```python
from build123d import *

# Parameters (mm, degrees)
F0_W     = 126
F0_H     = 129
F0_R     = 4
F1_DEPTH = 5


with BuildPart() as f1:
    # F0 (on Front) → F1 (new body)
    with BuildSketch(Plane.XZ):
        with Locations((63, 64.5)):
            Rectangle(F0_W, F0_H)
        with Locations((17, 27.5)):
            Circle(F0_R, mode=Mode.SUBTRACT)
        with Locations((17, 52.5)):
            Circle(F0_R, mode=Mode.SUBTRACT)
        with Locations((109, 27.5)):
            Circle(F0_R, mode=Mode.SUBTRACT)
        with Locations((109, 52.5)):
            Circle(F0_R, mode=Mode.SUBTRACT)
        with Locations((22, 107.5)):
            Circle(F0_R, mode=Mode.SUBTRACT)
        Polygon((93, 19), (33, 19), (24, 28), (24, 90), (49, 115), (77, 115), (102, 90), (102, 28), align=None, mode=Mode.SUBTRACT)
        with Locations((104, 107.5)):
            Circle(F0_R, mode=Mode.SUBTRACT)
    extrude(amount=F1_DEPTH)


solid = f1.part
```
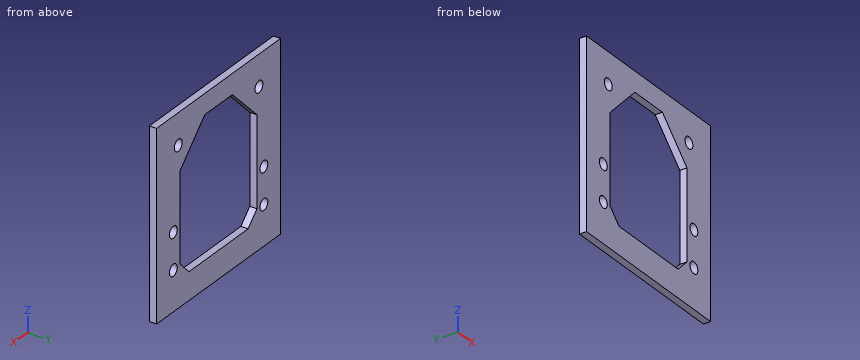
Design review of the part built by this model. Coordinates are the model's own, in mm. Round coordinates to 2 decimals unless told otherwise and drop trailing zeros. Write each loop counter-clockwise with the first axis right and the second up, starting at its lowest first coordinate (ties: lowest second). Pieces come first, ordered by that corner, then holes. Notation, with made-up numbers: (-2, -38.5) -> (53, -38.5) arc R18 ccw to (53, -18.5) -> close; hole circle Ø6 at (85.5, 11.5). An arc over 180 degrees is marked (long way). Answer in a Markdown table with one row per item.
Q1. To check wall thickness, follow L1, parallel to Z at x = 109, y = -2; L2, parallel to X at y = -2.15, z = 80.5; L3, parallel to Z at x = 36, y = -1.75. State the ranges of each line that lie inside material, in increasing order. Write a range as [from, to].
The answers:
| item | result |
|---|---|
| L1 | [0, 23.5], [31.5, 48.5], [56.5, 129] |
| L2 | [0, 24], [102, 126] |
| L3 | [0, 19], [102, 129] |
Q2. Take a section at D-D, the plane z = 38.5. State the section outline as (x, y) points, then the cut area to 3 significant figures.
The answers:
| item | result |
|---|---|
| outline | (0, -5) -> (24, -5) -> (24, 0) -> (0, 0) -> close; (102, -5) -> (126, -5) -> (126, 0) -> (102, 0) -> close |
| area | 240 mm² |
Q3. Take a section at B-B, the plane y = -0.9. State the section outline as (x, z) points.
The answers:
| item | result |
|---|---|
| outline | (0, 0) -> (126, 0) -> (126, 129) -> (0, 129) -> close; hole circle Ø8 at (17, 27.5); hole circle Ø8 at (17, 52.5); hole circle Ø8 at (22, 107.5); hole (24, 28) -> (33, 19) -> (93, 19) -> (102, 28) -> (102, 90) -> (77, 115) -> (49, 115) -> (24, 90) -> close; hole circle Ø8 at (104, 107.5); hole circle Ø8 at (109, 27.5); hole circle Ø8 at (109, 52.5) |
Q4. Take a section at A-A, the plane z = 107.5. State the section outline as (x, y) points.
The answers:
| item | result |
|---|---|
| outline | (0, -5) -> (18, -5) -> (18, 0) -> (0, 0) -> close; (26, -5) -> (41.5, -5) -> (41.5, 0) -> (26, 0) -> close; (84.5, -5) -> (100, -5) -> (100, 0) -> (84.5, 0) -> close; (108, -5) -> (126, -5) -> (126, 0) -> (108, 0) -> close |
Q5. Take a section at C-C, the plane x = 58. State the section outline as (y, z) points, then the cut area to 3 significant figures.
The answers:
| item | result |
|---|---|
| outline | (-5, 0) -> (0, 0) -> (0, 19) -> (-5, 19) -> close; (-5, 115) -> (0, 115) -> (0, 129) -> (-5, 129) -> close |
| area | 165 mm² |
